The drawing under review shows one solid part. Ordinate dimensions are in mm from its lowest x, y, z. A direction names the side the tool comes from. Coordinates: 2 decimals unless noted, no trailing zeros. Write each loop counter-clockwise with the first axis right and the second up, starting at its lowest first coordinate (ties: lowest second). Pieces come first, ordered by that corner, then holes. Notation, with made-up numbers: (31.5, -36.5) - (45.5, -36.5) arc R22 ccw to (45.5, -7.5) - close; hole circle Ø8 at (20.5, -14.75). An arc over 180 degrees is marked (long way). Put each result on its own line as item: value. Start each with the question number.
Item 1: Consider section D-D on y = 27.5. Give the boundary of the cut face in (x, z), then the cut area to 3 significant figures.
Item 2: Machinability: for the marked faces 1, 2, 3 and 4, which of the approach directions +Z, -Z, +X, -X, +Y, -Y give a long, thin tool a straight path to every point of the face, cutting with its end or side? Answer none if there is none.
Item 3: Consider section A-A on y = 23. Give the boundary of the cut face in (x, z), then the cut area to 3 significant figures.
Item 4: Consider section B-B on x = 20. Give the boundary of the cut face in (y, z).
Item 5: For pin 1 (7 mm diameter, centred on y = 10.5, z = 3, fed in from +X); pin 2 (6 mm diameter, centred on x = 33, y = 21.5, fed in from -Z); pin 3 (1 mm diameter, centred on y = 20, z = 26.5, fed in from -X); pin 4 (1 mm diameter, centred on y = 13.5, z = 15, fed in from +X), all flat-tipped, find the tip position at first contact; note any pin that passes through.
Item 6: To check wall thickness, follow L1, parallel to Y at x = 46, z = 2; L2, parallel to X at y = 14, z = 12; L3, parallel to X at y = 21.5, z = 10.5. State the ranges of each line that lie inside material, in increasing order. Write a range as [from, to].
Item 7: Consider section C-C on z = 3.5. Give the boundary of the cut face in (x, y).
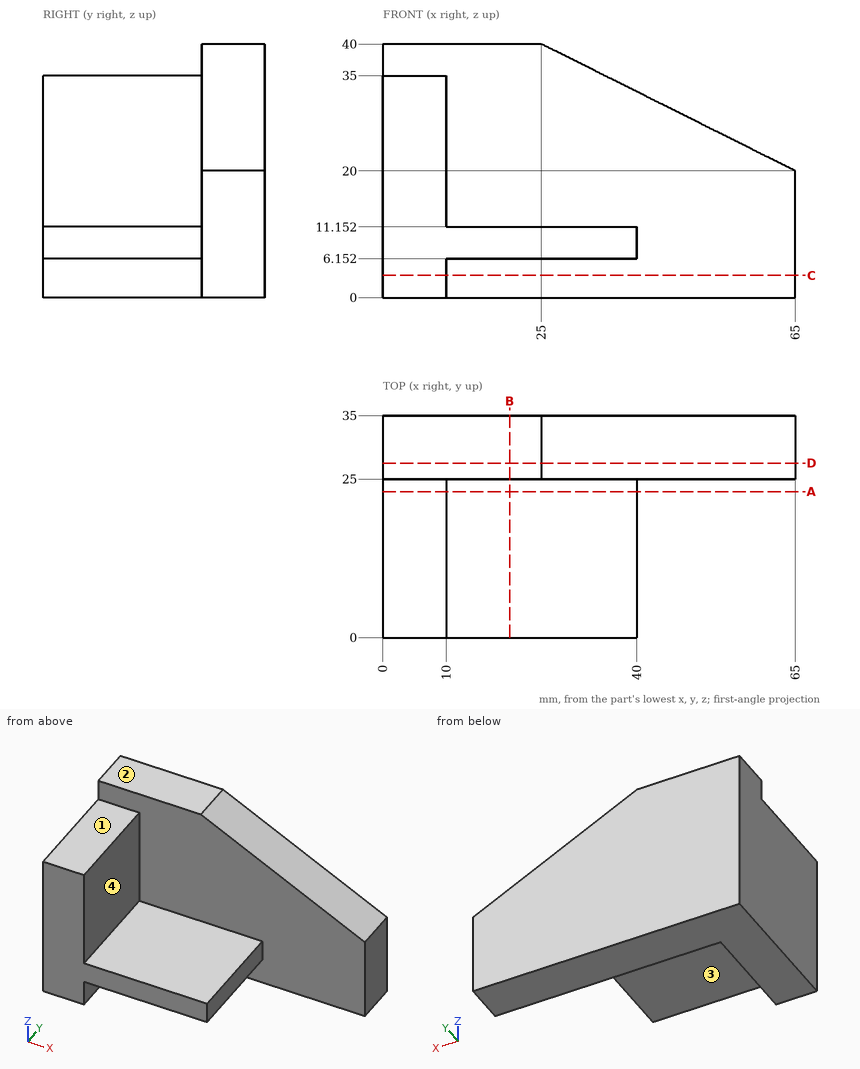
Report:
1. outline: (0, 0) - (65, 0) - (65, 20) - (25, 40) - (0, 40) - close
1. area: 2,200 mm²
2. face 1: +Z, +X, -X, -Y
2. face 2: +Z, +X, -X, +Y, -Y
2. face 3: -Z, +X, -Y
2. face 4: +Z, +X, -Y
3. outline: (0, 0) - (10, 0) - (10, 6.15) - (40, 6.15) - (40, 11.15) - (10, 11.15) - (10, 35) - (0, 35) - close
3. area: 500 mm²
4. outline: (0, 6.15) - (25, 6.15) - (25, 0) - (35, 0) - (35, 40) - (25, 40) - (25, 11.15) - (0, 11.15) - close
5. pin 1: x = 40
5. pin 2: z = 6.15
5. pin 3: x = 0
5. pin 4: x = 10
6. L1: [25, 35]
6. L2: [0, 10]
6. L3: [0, 40]
7. outline: (0, 0) - (10, 0) - (10, 25) - (65, 25) - (65, 35) - (0, 35) - close
